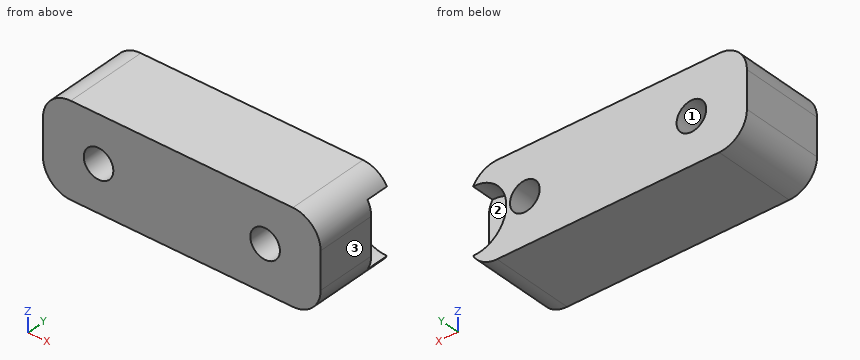
```python
from build123d import *

# Parameters (mm, degrees)
CYLINDER465_R     = 3.5
CYLINDER465_DEPTH = 2.5
CYLINDER152_R     = 1.6
CYLINDER152_DEPTH = 9
CYLINDER153_R     = 1.6
CYLINDER153_DEPTH = 9
CYLINDER154_R     = 1.6
CYLINDER154_DEPTH = 9
CYLINDER155_R     = 1.6
CYLINDER155_DEPTH = 9
BOX072_W          = 30
BOX072_H          = 9
BOX072_DEPTH      = 10
FILLET035_R       = 3


with BuildPart() as cylinder579:
    # Cylinder465 → Cylinder465 (new body)
    with BuildSketch(Plane(origin=(569.5, -10, 10), x_dir=(1, 0, 0), z_dir=(0, -1, 0))):
        Circle(CYLINDER465_R)
    extrude(amount=CYLINDER465_DEPTH)


with BuildPart() as cylinder152:
    # Cylinder152 → Cylinder152 (new body)
    with BuildSketch(Plane(origin=(555, -5, 10), x_dir=(1, 0, 0), z_dir=(0, -1, 0))):
        Circle(CYLINDER152_R)
    extrude(amount=CYLINDER152_DEPTH)


with BuildPart() as fusion138:
    # Cylinder153 → Cylinder153 (new body)
    with BuildSketch(Plane(origin=(450, -5, 10), x_dir=(1, 0, 0), z_dir=(0, -1, 0))):
        Circle(CYLINDER153_R)
    extrude(amount=CYLINDER153_DEPTH)

    # Fusion138: union Cylinder152
    add(cylinder152.part)


with BuildPart() as fusion138_1:
    # Fusion138 placement: moved
    add(fusion138.part.moved(Location((-9, 5, 0))))


with BuildPart() as cylinder154:
    # Cylinder154 → Cylinder154 (new body)
    with BuildSketch(Plane(origin=(555, -5, 10), x_dir=(1, 0, 0), z_dir=(0, -1, 0))):
        Circle(CYLINDER154_R)
    extrude(amount=CYLINDER154_DEPTH)


with BuildPart() as fusion137:
    # Cylinder155 → Cylinder155 (new body)
    with BuildSketch(Plane(origin=(450, -5, 10), x_dir=(1, 0, 0), z_dir=(0, -1, 0))):
        Circle(CYLINDER155_R)
    extrude(amount=CYLINDER155_DEPTH)

    # Fusion139: union Cylinder154
    add(cylinder154.part)


with BuildPart() as fusion137_1:
    # Fusion139 placement: moved
    add(fusion137.part.moved(Location((9, 5, 0))))

    # Fusion137: union Fusion138
    add(fusion138_1.part)


with BuildPart() as fender_spacer_rear_left:
    # Box072 → Box072 (new body)
    with BuildSketch(Plane(origin=(435, -9, 5), x_dir=(1, 0, 0), z_dir=(0, 0, 1))):
        with Locations((15, 4.5)):
            Rectangle(BOX072_W, BOX072_H)
    extrude(amount=BOX072_DEPTH)

    # Fillet035
    fillet035_edges = [fender_spacer_rear_left.edges().sort_by_distance(p)[0] for p in [
        (435, -4.5, 15),
        (435, -4.5, 5),
        (465, -4.5, 15),
        (465, -4.5, 5),
    ]]
    fillet(fillet035_edges, radius=FILLET035_R)


with BuildPart() as fender_spacer_rear_left_1:
    # Fillet035 placement: moved
    add(fender_spacer_rear_left.part.moved(Location((105, 0, 0))))

    # Cut082: cut Fusion137
    add(fusion137_1.part, mode=Mode.SUBTRACT)


with BuildPart() as fender_spacer_rear_left_2:
    # Cut082 placement: moved
    add(fender_spacer_rear_left_1.part.moved(Location((0, -10, 0))))

    # Cut321: cut Cylinder579
    add(cylinder579.part, mode=Mode.SUBTRACT)


solid = fender_spacer_rear_left_2.part
```
The listing builds one solid part. Answer for the finished solid, in the listing's coordinates (mm). Face numbers are marked on the shaded views. Give positions to 0.01 mm unless a question says otherwise; leave off trailing zeros. Order: outer loops, then holes, each group sorted by start corner. A loop starts at its lowest first (then second) coordinate and runs counter-clockwise, first axis right, second up. Notation, with made-up numbers: (42.5, -37) - (97.5, -37) arc R30 ccw to (97.5, -5) - close; hole circle Ø3 at (55.5, 26). An arc over 180 degrees is marked (long way). Use one line per item in the form item = value. Start each with the question number.
(1) A cutting plane is placed at C-C, the plane y = -18. Write down the section's boundary in (x, z).
(2) Consider line 1 (X direction, y = -16.75, z = 11); line 2 (Z direction, x = 564, y = -14.5); line 3 (X direction, y = -17.5, z = 11.25). Determine where each line is inside the solid, lowest interval first. Write a range as from..to.
(3) The mould has two halves that part along X. Classify the marked faces 1, 2 and 3: released by +X, released by -X, zero draft, split by the parting line, or undercut.
(4) A cutting plane is placed at B-B, the plane z = 10. Write down the section's boundary in (x, y).
(5) A cutting plane is placed at D-D, the plane x = 547. Write down the section's boundary in (y, z), then the cut area to 3 significant figures.
(6) A cutting plane is placed at A-A, the plane x = 564. Write down the section's boundary in (y, z).
Ans:
q1.outline = (540, 8) arc R3 ccw to (543, 5) - (567, 5) arc R3 ccw to (570, 8) - (570, 12) arc R3 ccw to (567, 15) - (543, 15) arc R3 ccw to (540, 12) - close; hole circle Ø3.2 at (546, 10); hole circle Ø3.2 at (564, 10)
q2.line_1 = 540..544.75, 547.25..562.75, 565.25..570
q2.line_2 = 5..8.4, 11.6..15
q2.line_3 = 540..545, 547..563, 565..570
q3.face_1 = undercut
q3.face_2 = zero draft
q3.face_3 = released by +X
q4.outline = (540, -19) - (544.4, -19) - (544.4, -10) - (540, -10) - close; (547.6, -19) - (562.4, -19) - (562.4, -10) - (547.6, -10) - close; (565.6, -19) - (570, -19) - (570, -12.5) - (566, -12.5) - (566, -10) - (565.6, -10) - close
q5.outline = (-19, 5) - (-10, 5) - (-10, 8.75) - (-19, 8.75) - close; (-19, 11.25) - (-10, 11.25) - (-10, 15) - (-19, 15) - close
q5.area = 67.5 mm^2
q6.outline = (-19, 5) - (-10, 5) - (-10, 8.4) - (-19, 8.4) - close; (-19, 11.6) - (-10, 11.6) - (-10, 15) - (-19, 15) - close
